Build history of the part. All positions in model axes, mm. Face numbers are marked on the shaded views. Round coordinates to 2 decimals unless told otherwise and drop trailing zeros. Write each loop counter-clockwise with the first axis right and the second up, starting at its lowest first coordinate (ties: lowest second). Pieces come first, ordered by that corner, then holes. Notation, with made-up numbers: (-33.5, -38) - (25.5, -38) arc R23 cw to (25.5, -9) - close; hole circle Ø5 at (-11, 0.25). An arc over 180 degrees is marked (long way). One line per question, with ' | ' between items.
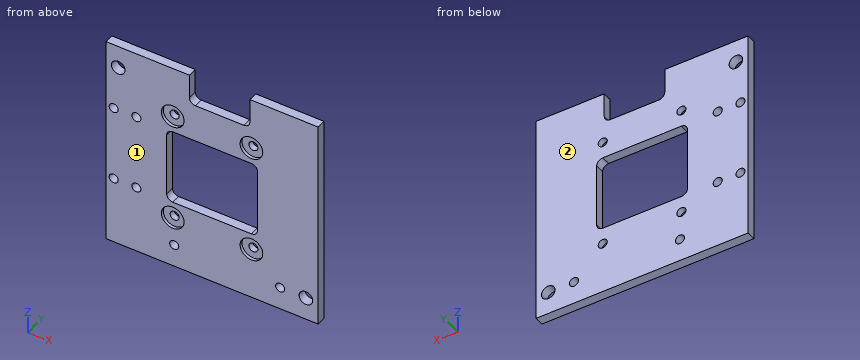
from build123d import *

# Parameters (mm, degrees)
F0_W     = 70
F0_H     = 70
F1_DEPTH = 3
F2_R     = 2.25
F2_R_2   = 1.5
F3_DEPTH = 3.001
F4_R     = 3.75
F5_DEPTH = 1
F6_R     = 1.5
F7_DEPTH = 3.001
F8_R     = 1.5
F9_DEPTH = 3.001


with BuildPart() as f1:
    # F0 (on Front) → F1 (new body)
    with BuildSketch(Plane.XZ):
        Rectangle(F0_W, F0_H)
    extrude(amount=F1_DEPTH)

    # F2 (on face) → F3 (cut, through all)
    with BuildSketch(Plane.XZ.offset(3)):
        with Locations((-31, 27.5)):
            Circle(F2_R)
        with Locations((31, -27.5)):
            Circle(F2_R)
        with Locations((-13, 18)):
            Circle(F2_R_2)
        with Locations((-13, -18)):
            Circle(F2_R_2)
        with Locations((13, 18)):
            Circle(F2_R_2)
        with Locations((13, -18)):
            Circle(F2_R_2)
        with BuildLine():
            Line((-13, -12.5), (13, -12.5))
            ThreePointArc((13, -12.5), (14.414214, -11.914214), (15, -10.5))
            Line((15, -10.5), (15, 10.5))
            ThreePointArc((15, 10.5), (14.414214, 11.914214), (13, 12.5))
            Line((13, 12.5), (-13, 12.5))
            ThreePointArc((-13, 12.5), (-14.414214, 11.914214), (-15, 10.5))
            Line((-15, 10.5), (-15, -10.5))
            ThreePointArc((-15, -10.5), (-14.414214, -11.914214), (-13, -12.5))
        make_face()
        with BuildLine():
            Line((12.5, 35), (-7.5, 35))
            Line((-7.5, 35), (-7.5, 27))
            ThreePointArc((-7.5, 27), (-6.914214, 25.585786), (-5.5, 25))
            Line((-5.5, 25), (10.5, 25))
            ThreePointArc((10.5, 25), (11.914214, 25.585786), (12.5, 27))
            Line((12.5, 27), (12.5, 35))
        make_face()
    extrude(amount=-F3_DEPTH, mode=Mode.SUBTRACT)

    # F4 (on face) → F5 (cut)
    with BuildSketch(Plane.XZ.offset(3)):
        with Locations((-13, 18)):
            Circle(F4_R)
        with Locations((13, 18)):
            Circle(F4_R)
        with Locations((-13, -18)):
            Circle(F4_R)
        with Locations((13, -18)):
            Circle(F4_R)
    extrude(amount=-F5_DEPTH, mode=Mode.SUBTRACT)

    # F6 (on face) → F7 (cut, through all)
    with BuildSketch(Plane.XZ.offset(3)):
        with Locations((-12.5, -27.5)):
            Circle(F6_R)
        with Locations((22.5, -27.5)):
            Circle(F6_R)
    extrude(amount=-F7_DEPTH, mode=Mode.SUBTRACT)

    # F8 (on face) → F9 (cut, through all)
    with BuildSketch(Plane.XZ.offset(3)):
        with Locations((-25, -12.5)):
            Circle(F8_R)
        with Locations((-25, 12.5)):
            Circle(F8_R)
        with Locations((-32.5, -12.5)):
            Circle(F8_R)
        with Locations((-32.5, 12.5)):
            Circle(F8_R)
    extrude(amount=-F9_DEPTH, mode=Mode.SUBTRACT)


solid = f1.part
Q1. Saw through at C-C, the plane z = -4. List the corners of the cut face in (x, y).
Found:
outline: (-35, -3) - (-15, -3) - (-15, 0) - (-35, 0) - close; (15, -3) - (35, -3) - (35, 0) - (15, 0) - close
Q2. Pull direction Y, two halves, no side cores. Call the marked faces 1 and 2: +Y half, -Y half, draft (parallel to the pull), parting line (faces both ways), or undercut.
Found:
face 1: -Y half | face 2: +Y half
Q3. Drill centre lines: L1, parallel to Z at x = -25, y = -1.05; L2, parallel to Z at x = 13, y = -2.5; L3, parallel to X at y = -1.9, z = 0. Where is each one in solid material? Low to high. Write a range as from..to.
Found:
L1: -35..-14, -11..11, 14..35 | L2: -35..-21.75, -14.25..-12.5, 12.5..14.25, 21.75..35 | L3: -35..-15, 15..35
Q4. Drop flat-ended pins along their axis: pin 1 (2.5 mm diameter, centred on x = -32.5, z = -12.5, fed in from +Y); pin 2 (0.9 mm diameter, centred on x = -1, y = -1, fed in from +Z); pin 3 (3.5 mm diameter, centred on x = 13, z = 18, fed in from -Y). Give the stop position or say it passes through.
Found:
pin 1: through | pin 2: z = 25 | pin 3: y = -2
Q5. Saw through at B-B, the plane x = 31. List the corners of the cut face in (y, z).
Found:
outline: (-3, -35) - (0, -35) - (0, -29.75) - (-3, -29.75) - close; (-3, -25.25) - (0, -25.25) - (0, 35) - (-3, 35) - close
Q6. Saw through at A-A, the plane y = -1.35. State how many separate pieces and enclosed holes the cut face has, then the cut area to 3 significant figures.
Found:
separate pieces: 1 | enclosed holes: 13 | area: 3,850 mm^2
